Input: part model. Units: mm. Frame: model coordinates. Face numbers are marked on the shaded views. A direction names the side the tool comes from. Give positions to 0.01 mm unless a question says otherwise; leave off trailing zeros. Loops run counter-clockwise (first coordinate to the right, second up) from the corner with the lowest first, then second, coordinate; pieces in that order, holes last.
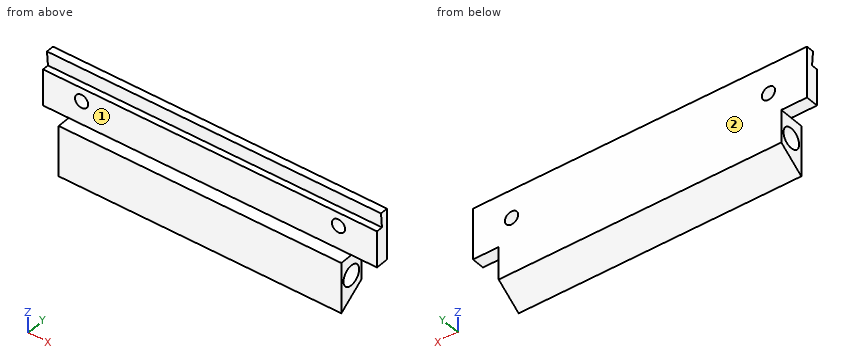
from build123d import *

# Parameters (mm, degrees)
F0_W         = 165.1
F0_H         = 38.1
F1_DEPTH     = 12.7
F3_DEPTH     = 165.101
F4_W         = 165.1
F4_H         = 12.7
F5_DEPTH     = 12.7
F7_D         = 6.5278
F9_W         = 12.7
F9_H         = 25.4
F10_DEPTH    = 12.701
F11_D        = 9.9314
F12_T1_DEPTH = 207.1510236039


# Not quite as in the source:
# - a fillet or chamfer that OpenCascade refuses, or shapes differently, is made with other operations: its cross-section is extruded or revolved along the edge and cut away or added


with BuildPart() as f1:
    # F0 (on Front) → F1 (new body)
    with BuildSketch(Plane.XZ):
        with Locations((82.55, 19.05)):
            Rectangle(F0_W, F0_H)
    extrude(amount=F1_DEPTH)

    # F2 (on face) → F3 (cut, through all)
    with BuildSketch(Plane.YZ.offset(165.1)):
        Polygon((-6.35, 12.7), (-6.35, 30.734), (-3.2131, 30.734), (-3.81, 38.1), (-8.89, 38.1), (-12.7, 38.1), (-12.7, 27.7622), (-12.7, 12.7), align=None)
    extrude(amount=-F3_DEPTH, mode=Mode.SUBTRACT)

    # F4 (on face) → F5 (join)
    with BuildSketch(Plane.XZ.offset(12.7)):
        with Locations((82.55, -6.35)):
            Rectangle(F4_W, F4_H)
    extrude(amount=-F5_DEPTH)

    # F7 (through all)
    with Locations(Plane.XZ.offset(6.35)):
        with Locations((19.05, 24.13), (146.05, 24.13)):
            Hole(F7_D / 2)

    # F9 (on face) → F10 (cut, through all)
    with BuildSketch(Plane.XZ.offset(12.7)):
        with Locations((6.35, 0)):
            Rectangle(F9_W, F9_H)
        with Locations((158.75, 0)):
            Rectangle(F9_W, F9_H)
    extrude(amount=-F10_DEPTH, mode=Mode.SUBTRACT)

    # F11 (through all)
    with Locations(Plane(origin=(0, 0, 0), x_dir=(0, -1, 0), z_dir=(-1, 0, 0))):
        with Locations((6.35, 2.54)):
            Hole(F11_D / 2)

    # F12: chamfer of 9.144 x 13.0589853736 on 1 edges, made by hand

    # F12_s2 → F12_t1 (cut)
    with BuildSketch(Plane.YZ.offset(-21.025511802)):
        Polygon((0, -3.556), (-13.0589853736, -12.7), (0, -12.7), align=None)
    extrude(amount=F12_T1_DEPTH, mode=Mode.SUBTRACT)


solid = f1.part
(1) Ray query, probe 1 along Z at (x, y) = (146.05, -2.5); probe 2 along Y at (x, z) = (65, 3); probe 3 along X at (y, z) = (-10.75, -1). Return the intervals inside material, ascending.
Values follow:
probe 1: z = -5.31 to -0.6, 5.68 to 20.87, 27.39 to 38.1
probe 2: y = -12.7 to -11.29, -1.41 to 0
probe 3: x = 12.7 to 152.4
(2) Cut plane D-D (x = 74). Return the cut outline in (y, z).
Values follow:
outline: (-12.7, -12.45) - (0, -3.56) - (0, 38.1) - (-3.81, 38.1) - (-3.21, 30.73) - (-6.35, 30.73) - (-6.35, 12.7) - (-12.7, 12.7) - close; hole circle Ø9.93 at (-6.35, 2.54)
(3) Cut plane A-A (x = 19.05). Return the cut outline in (y, z), and give its area (3 significant figures).
Values follow:
outline: (-12.7, -12.45) - (0, -3.56) - (0, 20.87) - (-6.35, 20.87) - (-6.35, 12.7) - (-12.7, 12.7) - close; (-6.35, 27.39) - (0, 27.39) - (0, 38.1) - (-3.81, 38.1) - (-3.21, 30.73) - (-6.35, 30.73) - close; hole circle Ø9.93 at (-6.35, 2.54)
area: 284 mm2
(4) Reachability of the marked faces 1 and 2 from +Z, -Z, +X, -X, +Y, -Y: full face, straight path, thin tool, end or side. Return the list, or none.
Values follow:
face 1: +Z, +X, -X, -Y
face 2: +Z, -Z, +X, -X, +Y
(5) Pin query (flat end, axial travel): pin 1 Ø9 at (x, z) = (119, 20.5) entering from -Y; pin 2 Ø2 at (x, y) = (82.5, -3) entering from -Z; pin 3 Ø7 at (x, y) = (8, -3.5) entering from -Z; pin 4 Ø5 at (x, z) = (19.05, 24.13) entering from -Y. Return the tip coordinate at first contact, or that it passes through.
Values follow:
pin 1: stops at y = -6.35
pin 2: stops at z = -6.36
pin 3: stops at z = 12.7
pin 4: passes through
(6) Cut plane C-C (z = 24.13). Return the cut outline in (x, y), and give its area (3 significant figures).
Values follow:
outline: (0, -6.35) - (15.79, -6.35) - (15.79, 0) - (0, 0) - close; (22.31, -6.35) - (142.79, -6.35) - (142.79, 0) - (22.31, 0) - close; (149.31, -6.35) - (165.1, -6.35) - (165.1, 0) - (149.31, 0) - close
area: 965 mm2
(7) Cut plane B-B (z = 2.54). Return the cut outline in (x, y).
Values follow:
outline: (12.7, -12.7) - (152.4, -12.7) - (152.4, -11.32) - (12.7, -11.32) - close; (12.7, -1.38) - (152.4, -1.38) - (152.4, 0) - (12.7, 0) - close
